Input: part model. Units: mm. Frame: model coordinates. A direction names the side the tool comes from. Give positions to 0.01 mm unless a question says otherwise; leave off trailing zeros. Order: outer loops, then holes, each group sorted by start corner. A loop starts at its lowest first (then second) coordinate and runs counter-clockwise, first axis right, second up. Notation, with made-up numbers: M 84.5,-25 L 91.5,-25 A24 cw 91.5,-8 Z; hole C -34.75,-33 d6. An arc over 180 degrees is marked long. Use a Markdown table: item, result.
from build123d import *

# Parameters (mm, degrees)
CROQUIS1_R               = 65
SALIENTE_EXTRUIR2_DEPTH  = 35
CROQUIS2_R               = 13.5
SALIENTE_EXTRUIR3_DEPTH  = 400
CROQUIS3_R               = 13.5
SALIENTE_EXTRUIR4_DEPTH  = 10.5
CROQUIS4_R               = 13.5
SALIENTE_EXTRUIR6_DEPTH  = 10.5
CROQUIS5_R               = 13.5
SALIENTE_EXTRUIR7_DEPTH  = 10.5
CROQUIS6_R               = 13.5
SALIENTE_EXTRUIR8_DEPTH  = 10.5
CROQUIS7_R               = 13.5
SALIENTE_EXTRUIR9_DEPTH  = 10.5
CROQUIS8_R               = 13.5
SALIENTE_EXTRUIR10_DEPTH = 10.5
CROQUIS9_R               = 13.5
SALIENTE_EXTRUIR11_DEPTH = 10.5
CROQUIS10_R              = 13.5
SALIENTE_EXTRUIR12_DEPTH = 10.5
SALIENTE_EXTRUIR13_DEPTH = 32.7
SALIENTE_EXTRUIR14_DEPTH = 31.9
SALIENTE_EXTRUIR15_DEPTH = 31.9
SALIENTE_EXTRUIR16_DEPTH = 31.9


with BuildPart() as part:
    # Croquis1 → Saliente-Extruir2 (new body)
    with BuildSketch(Plane.XY):
        Circle(CROQUIS1_R)
    extrude(amount=SALIENTE_EXTRUIR2_DEPTH)

    # Croquis2 → Saliente-Extruir3 (add)
    with BuildSketch(Plane.XY.offset(35)):
        Circle(CROQUIS2_R)
    extrude(amount=SALIENTE_EXTRUIR3_DEPTH)

    # Croquis3 → Saliente-Extruir4 (add)
    with BuildSketch(Plane.XY.offset(392.6)):
        with BuildLine():
            Line((-19.616978627, 15.497553018), (-4.708074871, 34.369412724))
            ThreePointArc((-4.708074871, 34.369412724), (0, 36.65), (4.708074871, 34.369412724))
            Line((4.708074871, 34.369412724), (19.616978627, 15.497553018))
            ThreePointArc((19.616978627, 15.497553018), (0, -25), (-19.616978627, 15.497553018))
        make_face()
        Circle(CROQUIS3_R, mode=Mode.SUBTRACT)
    extrude(amount=SALIENTE_EXTRUIR4_DEPTH)

    # Croquis4 → Saliente-Extruir6 (add)
    with BuildSketch(Plane.XY.offset(349.4)):
        with BuildLine():
            Line((18.668562955, 16.627830803), (34.664812739, -1.331637253))
            ThreePointArc((34.664812739, -1.331637253), (36.093204148, -6.364205711), (33.029715496, -10.604734521))
            Line((33.029715496, -10.604734521), (11.855657775, -22.010074483))
            ThreePointArc((11.855657775, -22.010074483), (-24.620193825, 4.341204442), (18.668562955, 16.627830803))
        make_face()
        Circle(CROQUIS4_R, mode=Mode.SUBTRACT)
    extrude(amount=SALIENTE_EXTRUIR6_DEPTH)

    # Croquis5 → Saliente-Extruir7 (add)
    with BuildSketch(Plane.XY.offset(307)):
        with BuildLine():
            Line((-15.497553018, -19.616978627), (-34.369412724, -4.708074871))
            ThreePointArc((-34.369412724, -4.708074871), (-36.65, 0), (-34.369412724, 4.708074871))
            Line((-34.369412724, 4.708074871), (-15.497553018, 19.616978627))
            ThreePointArc((-15.497553018, 19.616978627), (25, 0), (-15.497553018, -19.616978627))
        make_face()
        Circle(CROQUIS5_R, mode=Mode.SUBTRACT)
    extrude(amount=SALIENTE_EXTRUIR7_DEPTH)

    # Croquis6 → Saliente-Extruir8 (add)
    with BuildSketch(Plane.XY.offset(264.6)):
        with BuildLine():
            Line((-16.627830803, 18.668562955), (1.331637253, 34.664812739))
            ThreePointArc((1.331637253, 34.664812739), (6.364205711, 36.093204148), (10.604734521, 33.029715496))
            Line((10.604734521, 33.029715496), (22.010074483, 11.855657775))
            ThreePointArc((22.010074483, 11.855657775), (-4.341204442, -24.620193825), (-16.627830803, 18.668562955))
        make_face()
        Circle(CROQUIS6_R, mode=Mode.SUBTRACT)
    extrude(amount=SALIENTE_EXTRUIR8_DEPTH)

    # Croquis7 → Saliente-Extruir9 (add)
    with BuildSketch(Plane.XY.offset(222.2)):
        with BuildLine():
            Line((16.627830803, -18.668562955), (-1.331637253, -34.664812739))
            ThreePointArc((-1.331637253, -34.664812739), (-6.364205711, -36.093204148), (-10.604734521, -33.029715496))
            Line((-10.604734521, -33.029715496), (-22.010074483, -11.855657775))
            ThreePointArc((-22.010074483, -11.855657775), (4.341204442, 24.620193825), (16.627830803, -18.668562955))
        make_face()
        Circle(CROQUIS7_R, mode=Mode.SUBTRACT)
    extrude(amount=SALIENTE_EXTRUIR9_DEPTH)

    # Croquis8 → Saliente-Extruir10 (add)
    with BuildSketch(Plane.XY.offset(179.8)):
        with BuildLine():
            Line((15.497553018, 19.616978627), (34.369412724, 4.708074871))
            ThreePointArc((34.369412724, 4.708074871), (36.65, 0), (34.369412724, -4.708074871))
            Line((34.369412724, -4.708074871), (15.497553018, -19.616978627))
            ThreePointArc((15.497553018, -19.616978627), (-25, 0), (15.497553018, 19.616978627))
        make_face()
        Circle(CROQUIS8_R, mode=Mode.SUBTRACT)
    extrude(amount=SALIENTE_EXTRUIR10_DEPTH)

    # Croquis9 → Saliente-Extruir11 (add)
    with BuildSketch(Plane.XY.offset(137.4)):
        with BuildLine():
            Line((-18.668562955, -16.627830803), (-34.664812739, 1.331637253))
            ThreePointArc((-34.664812739, 1.331637253), (-36.093204148, 6.364205711), (-33.029715496, 10.604734521))
            Line((-33.029715496, 10.604734521), (-11.855657775, 22.010074483))
            ThreePointArc((-11.855657775, 22.010074483), (24.620193825, -4.341204442), (-18.668562955, -16.627830803))
        make_face()
        Circle(CROQUIS9_R, mode=Mode.SUBTRACT)
    extrude(amount=SALIENTE_EXTRUIR11_DEPTH)

    # Croquis10 → Saliente-Extruir12 (add)
    with BuildSketch(Plane.XY.offset(95)):
        with BuildLine():
            Line((19.616978627, -15.497553018), (4.708074871, -34.369412724))
            ThreePointArc((4.708074871, -34.369412724), (0, -36.65), (-4.708074871, -34.369412724))
            Line((-4.708074871, -34.369412724), (-19.616978627, -15.497553018))
            ThreePointArc((-19.616978627, -15.497553018), (0, 25), (19.616978627, -15.497553018))
        make_face()
        Circle(CROQUIS10_R, mode=Mode.SUBTRACT)
    extrude(amount=SALIENTE_EXTRUIR12_DEPTH)

    # Croquis11 → Saliente-Extruir13 (add)
    with BuildSketch(Plane.XY.offset(359.9)):
        with BuildLine():
            Line((-5.302212899, 20.117414279), (11.86301125, 17.090722131))
            ThreePointArc((11.86301125, 17.090722131), (15.45729222, 15.703316474), (18.260288087, 13.060029823))
            ThreePointArc((18.260288087, 13.060029823), (-3.898401589, -22.108934055), (-12.692264697, 18.517800001))
            ThreePointArc((-12.692264697, 18.517800001), (-9.154252885, 20.042995913), (-5.302212899, 20.117414279))
        make_face()
    extrude(amount=SALIENTE_EXTRUIR13_DEPTH)

    # Croquis12 → Saliente-Extruir14 (add)
    with BuildSketch(Plane.XY.offset(275.1)):
        with BuildLine():
            Line((-20.117414279, -5.302212899), (-17.090722131, 11.86301125))
            ThreePointArc((-17.090722131, 11.86301125), (-15.703316474, 15.45729222), (-13.060029823, 18.260288087))
            ThreePointArc((-13.060029823, 18.260288087), (22.108934055, -3.898401589), (-18.517800001, -12.692264697))
            ThreePointArc((-18.517800001, -12.692264697), (-20.042995913, -9.154252885), (-20.117414279, -5.302212899))
        make_face()
    extrude(amount=SALIENTE_EXTRUIR14_DEPTH)

    # Croquis14 → Saliente-Extruir15 (add)
    with BuildSketch(Plane.XY.offset(190.3)):
        with BuildLine():
            Line((20.117414279, 5.302212899), (17.090722131, -11.86301125))
            ThreePointArc((17.090722131, -11.86301125), (15.703316474, -15.45729222), (13.060029823, -18.260288087))
            ThreePointArc((13.060029823, -18.260288087), (-22.108934055, 3.898401589), (18.517800001, 12.692264697))
            ThreePointArc((18.517800001, 12.692264697), (20.042995913, 9.154252885), (20.117414279, 5.302212899))
        make_face()
    extrude(amount=SALIENTE_EXTRUIR15_DEPTH)

    # Croquis15 → Saliente-Extruir16 (add)
    with BuildSketch(Plane.XY.offset(105.5)):
        with BuildLine():
            Line((-5.302212899, 20.117414279), (11.86301125, 17.090722131))
            ThreePointArc((11.86301125, 17.090722131), (15.45729222, 15.703316474), (18.260288087, 13.060029823))
            ThreePointArc((18.260288087, 13.060029823), (-3.898401589, -22.108934055), (-12.692264697, 18.517800001))
            ThreePointArc((-12.692264697, 18.517800001), (-9.154252885, 20.042995913), (-5.302212899, 20.117414279))
        make_face()
    extrude(amount=SALIENTE_EXTRUIR16_DEPTH)


solid = part.part
1) Material intervals for line 1 (Z direction, x = 14, y = -2); line 2 (Z direction, x = -20.5, y = 1); line 3 (Z direction, x = 10, y = 30), sorted ascending. Write a range as from..to.
Response values:
| item | result |
|---|---|
| line 1 | z = 0..35, 95..147.9, 179.8..232.7, 264.6..317.5, 349.4..403.1 |
| line 2 | z = 0..35, 95..147.9, 179.8..232.7, 264.6..275.1, 307..317.5, 349.4..403.1 |
| line 3 | z = 0..35, 264.6..275.1 |
2) Cut plane C-C on z = 68.5. Return loops of the section in (x, y), and give its area (3 significant figures).
Response values:
| item | result |
|---|---|
| outline | C 0,0 d27 |
| area | 573 mm² |
3) Reachability of faces 4 (the face through (-2.93, -13.18, 418.83)), 5 (the face through (-18.625, 3.16, 290.827)), 6 (the face through (-11, -12, 95)) from +Z, -Z, +X, -X, +Y, -Y: full face, straight path, thin tool, end or side. Return the list, or none.
Response values:
| item | result |
|---|---|
| face 4 | +Z |
| face 5 | -X, +Y |
| face 6 | none |
4) Cut plane B-B on y = -46.5. Return loops of the section in (x, z).
Response values:
| item | result |
|---|---|
| outline | M -45.42,0 L 45.42,0 L 45.42,35 L -45.42,35 Z |
5) Mould query, pull axis Z, two halves, no side actions, for faces 1 (the face through (-1, 1, 0)), 2 (the face through (-2.93, -13.18, 248.43)), 3 (the face through (-12.27, 24.8, 397.78)). Classes: released by +Z, released by -Z, zero draft, split by the parting line, or undercut.
Response values:
| item | result |
|---|---|
| face 1 | released by -Z |
| face 2 | undercut |
| face 3 | zero draft |
6) Cut plane A-A on z = 301. Return loops of the section in (x, y), and give its area (3 significant figures).
Response values:
| item | result |
|---|---|
| outline | M -20.12,-5.3 A10 ccw -18.52,-12.69 A22.45 ccw long -13.06,18.26 A10 ccw -17.09,11.86 Z |
| area | 1,520 mm² |
7) First-contact query: pin 1 Ø10 at (y, z) = (17, 275) entering from +X; pin 2 Ø8 at (y, z) = (7, 94) entering from +X; pin 3 Ø1 at (x, z) = (10, 44.5) entering from -Y. Flat tips, straight axial feed; report the tip coordinate or a pass-through.
Response values:
| item | result |
|---|---|
| pin 1 | stops at x = 21.93 |
| pin 2 | stops at x = 24.8 |
| pin 3 | stops at y = -9.59 |
